```python
from build123d import *

# Parameters (mm, degrees)
BOSS_EXTRUDE1_DEPTH      = 35
BOSS_EXTRUDE1_DEPTH_BACK = 35


with BuildPart() as part:
    # Sketch1 → Boss-Extrude1 (new, two sides: drawn at the far end of the back side and taken through both)
    with BuildSketch(Plane.XY.offset(-BOSS_EXTRUDE1_DEPTH_BACK)):
        with BuildLine():
            Line((-15, 5.25), (-15, -5.25))
            ThreePointArc((-15, -5.25), (-14.707106781, -5.957106781), (-14, -6.25))
            Line((-14, -6.25), (14, -6.25))
            ThreePointArc((14, -6.25), (14.707106781, -5.957106781), (15, -5.25))
            Line((15, -5.25), (15, 5.25))
            ThreePointArc((15, 5.25), (14.707106781, 5.957106781), (14, 6.25))
            Line((14, 6.25), (6.6, 6.25))
            ThreePointArc((6.6, 6.25), (6.246446609, 6.103553391), (6.1, 5.75))
            Line((6.1, 5.75), (6.1, 3.45))
            ThreePointArc((6.1, 3.45), (6.158578644, 3.308578644), (6.3, 3.25))
            Line((6.3, 3.25), (10, 3.25))
            ThreePointArc((10, 3.25), (10.707106781, 2.957106781), (11, 2.25))
            Line((11, 2.25), (11, -2.25))
            ThreePointArc((11, -2.25), (10.707106781, -2.957106781), (10, -3.25))
            Line((10, -3.25), (-10, -3.25))
            ThreePointArc((-10, -3.25), (-10.707106781, -2.957106781), (-11, -2.25))
            Line((-11, -2.25), (-11, 2.25))
            ThreePointArc((-11, 2.25), (-10.707106781, 2.957106781), (-10, 3.25))
            Line((-10, 3.25), (-6.3, 3.25))
            ThreePointArc((-6.3, 3.25), (-6.158578644, 3.308578644), (-6.1, 3.45))
            Line((-6.1, 3.45), (-6.1, 5.75))
            ThreePointArc((-6.1, 5.75), (-6.246446609, 6.103553391), (-6.6, 6.25))
            Line((-6.6, 6.25), (-14, 6.25))
            ThreePointArc((-14, 6.25), (-14.707106781, 5.957106781), (-15, 5.25))
        make_face()
    extrude(amount=BOSS_EXTRUDE1_DEPTH + BOSS_EXTRUDE1_DEPTH_BACK)

    # Sketch2 → Cut-Revolve1 (revolve, cut)
    with BuildSketch(Plane(origin=(0, 0, 0), x_dir=(0, 0, -1), z_dir=(1, 0, 0)), mode=Mode.PRIVATE) as cut_revolve1_sk:
        Polygon((-20, -3.25), (-17, -3.25), (-17, -5.25), (-18.25, -5.25), (-18.25, -6.25), (-20, -6.25), align=None)
    revolve(cut_revolve1_sk.sketch.rotate(Axis((0, -6.25, 20), (0, 1, 0)), 180), axis=Axis((0, -6.25, 20), (0, 1, 0)), mode=Mode.SUBTRACT)

    # Sketch3 → Cut-Revolve2 (revolve, cut)
    with BuildSketch(Plane(origin=(0, 0, 0), x_dir=(0, 0, -1), z_dir=(1, 0, 0)), mode=Mode.PRIVATE) as cut_revolve2_sk:
        Polygon((20, -3.25), (23, -3.25), (23, -5.25), (21.75, -5.25), (21.75, -6.25), (20, -6.25), align=None)
    revolve(cut_revolve2_sk.sketch.rotate(Axis((0, -6.25, -20), (0, 1, 0)), 180), axis=Axis((0, -6.25, -20), (0, 1, 0)), mode=Mode.SUBTRACT)


solid = part.part
```
Check sheet for the modelled part. Datum: model origin and axes. Units: mm. A direction names the side the tool comes from. Round coordinates to 2 decimals unless told otherwise and drop trailing zeros. Loops run counter-clockwise (first coordinate to the right, second up) from the corner with the lowest first, then second, coordinate; pieces in that order, holes last. Notation, with made-up numbers: (27, 40) -> (53, 40) arc R18 cw to (53, 71) -> close; hole circle Ø3 at (-18, 88.25). An arc over 180 degrees is marked (long way). Write item = value, one per line. Start each with the question number.
1) Sectioned sample at C-C, the plane y = -0.25. Record the cut outline in (x, z).
2) Thickness scan on probe 1 along X at (y, z) = (-0.25, 26.5); probe 2 along X at (y, z) = (3.5, -25); probe 3 along Y at (x, z) = (-7.5, -28). Record the ranges inside material, lowest first.
3) Sectioned sample at B-B, the plane x = -8.5. Record the cut outline in (y, z).
4) Sectioned sample at D-D, the plane x = 0. Record the cut outline in (y, z).
5) Set-up check for faces 5 (the flat face through (-15, 0, 0)), 6 (the flat face through (-11, 0, 0)), 7 (the flat face through (-6.1, 5, 0)), 8 (the cylindrical face through (0.08, -5.76, 18.25)), 9 (the flat face through (-2, -5.25, 20)): record each of +Z, -Z, +X, -X, +Y, -Y from which the full face is reachable in a straight line by a thin tool's end or side.
6) Gauge pin test, flat ends, axial feed: pin 1 Ø5.5 at (x, z) = (0, -20) entering from +Y; pin 2 Ø5 at (x, z) = (0, 21) entering from +Y. Record the tip position at first contact, or that the pin passes through.
7) Release check for a two-part mould opening along Z. For faces 1 (the cylindrical face through (0, -4, -23)), 2 (the cylindrical face through (0.08, -5.76, -21.75)), 3 (the flat face through (10, 6.25, 0)), 4 (the flat face through (0, -4, -35)) record: released by +Z, released by -Z, zero draft, split by the parting line, or undercut.
Results are:
q1.outline = (-15, -35) -> (-11, -35) -> (-11, 35) -> (-15, 35) -> close; (11, -35) -> (15, -35) -> (15, 35) -> (11, 35) -> close
q2.probe_1 = -15 to -11, 11 to 15
q2.probe_2 = -15 to -6.1, 6.1 to 15
q2.probe_3 = -6.25 to -3.25, 3.25 to 6.25
q3.outline = (-6.25, -35) -> (-3.25, -35) -> (-3.25, 35) -> (-6.25, 35) -> close; (3.25, -35) -> (6.25, -35) -> (6.25, 35) -> (3.25, 35) -> close
q4.outline = (-6.25, -35) -> (-3.25, -35) -> (-3.25, -23) -> (-5.25, -23) -> (-5.25, -21.75) -> (-6.25, -21.75) -> close; (-6.25, -18.25) -> (-5.25, -18.25) -> (-5.25, -17) -> (-3.25, -17) -> (-3.25, 17) -> (-5.25, 17) -> (-5.25, 18.25) -> (-6.25, 18.25) -> close; (-6.25, 21.75) -> (-5.25, 21.75) -> (-5.25, 23) -> (-3.25, 23) -> (-3.25, 35) -> (-6.25, 35) -> close
q5.face_5 = +Z, -Z, -X, +Y, -Y
q5.face_6 = +Z, -Z
q5.face_7 = +Z, -Z, +Y
q5.face_8 = +Y, -Y
q5.face_9 = +Y
q6.pin_1 = -5.25
q6.pin_2 = -3.25
q7.face_1 = undercut
q7.face_2 = undercut
q7.face_3 = zero draft
q7.face_4 = released by -Z
